Work out the finished part from the listing and answer in its coordinate system (mm). Round coordinates to 2 decimals unless told otherwise and drop trailing zeros. Order: outer loops, then holes, each group sorted by start corner. A loop starts at its lowest first (then second) coordinate and runs counter-clockwise, first axis right, second up. Notation, with made-up numbers: (-29, 7.25) -> (25, 7.25) arc R29 cw to (25, 37.25) -> close; hole circle Ø7 at (41, 0.5). An arc over 180 degrees is marked (long way). Use a Markdown table: item, result. Add a question column.
Item 1: Find the intervals of material crossed by L1, parallel to Z at x = 9, y = 1.85; L2, parallel to X at y = 0.75, z = 5.5; L3, parallel to X at y = -1.1, z = -5, in increasing order. Write a range as [from, to].
Item 2: A cutting plane is placed at D-D, the plane x = -34.7. Determine the outline of the cut face in (y, z), plus the area to 3 significant figures.
Item 3: A cutting plane is placed at A-A, the plane x = -23. Determine the outline of the cut face in (y, z).
Item 4: A cutting plane is placed at B-B, the plane z = 5. Determine the outline of the cut face in (x, y), plus the area to 3 significant figures.
Item 5: A cutting plane is placed at C-C, the plane z = -17.5. Determine the outline of the cut face in (x, y), plus the area to 3 significant figures.
Item 6: Flat-ended cylindrical pins translate along their axes: P1, Ø0.9, axis at y = -1, z = -15.5, coming from the -X side; P2, Ø1.5, axis at y = -1, z = -28, coming from the -X side; P3, Ø2, axis at x = 19, y = -1, coming from the -Z side. Find the tip coordinate at first contact, or state that the pin passes through.
from build123d import *

# Parameters (mm, degrees)
ESTRUSIONE_ESTRUSIONE1_DEPTH = 2
CORTAR_EXTRUIR4_DEPTH        = 10
CROQUIS2_R                   = 2
CROQUIS2_W                   = 40.7
CROQUIS2_H                   = 20
CORTAR_EXTRUIR5_DEPTH        = 59.660037504


with BuildPart() as part:
    # Schizzo1 → Estrusione-Estrusione1 (new, symmetric)
    with BuildSketch(Plane(origin=(0, 0, 0), x_dir=(1, 0, 0), z_dir=(0, 1, 0))):
        with BuildLine():
            Line((-25, 37.416573868), (-25, 27.25))
            Line((-25, 27.25), (25, 27.25))
            Line((25, 27.25), (25, 37.416573868))
            ThreePointArc((25, 37.416573868), (45, 0), (25, -37.416573868))
            Line((25, -37.416573868), (25, -27.25))
            Line((25, -27.25), (-25, -27.25))
            Line((-25, -27.25), (-25, -37.416573868))
            ThreePointArc((-25, -37.416573868), (-45, 0), (-25, 37.416573868))
        make_face()
    extrude(amount=ESTRUSIONE_ESTRUSIONE1_DEPTH, both=True)

    # Croquis1 → Cortar-Extruir4 (cut)
    with BuildSketch(Plane.XZ.offset(2)):
        Polygon((-8.5, 27.25), (-11.5, 27.25), (-11.5, 19.25), (-12.75, 19.25), (-12.75, 16.25), (-11.5, 16.25), (-11.5, 13.25), (-8.5, 13.25), (-8.5, 16.25), (-7.25, 16.25), (-7.25, 19.25), (-8.5, 19.25), align=None)
        Polygon((11.5, 27.25), (8.5, 27.25), (8.5, 19.25), (7.25, 19.25), (7.25, 16.25), (8.5, 16.25), (8.5, 13.25), (11.5, 13.25), (11.5, 16.25), (12.75, 16.25), (12.75, 19.25), (11.5, 19.25), align=None)
        Polygon((8.5, -13.25), (8.5, -16.25), (7.25, -16.25), (7.25, -19.25), (8.5, -19.25), (8.5, -27.25), (11.5, -27.25), (11.5, -19.25), (12.75, -19.25), (12.75, -16.25), (11.5, -16.25), (11.5, -13.25), align=None)
        Polygon((-11.5, -13.25), (-11.5, -16.25), (-12.75, -16.25), (-12.75, -19.25), (-11.5, -19.25), (-11.5, -27.25), (-8.5, -27.25), (-8.5, -19.25), (-7.25, -19.25), (-7.25, -16.25), (-8.5, -16.25), (-8.5, -13.25), align=None)
    extrude(amount=-CORTAR_EXTRUIR4_DEPTH, mode=Mode.SUBTRACT)

    # Croquis2 → Cortar-Extruir5 (cut, through all)
    with BuildSketch(Plane(origin=(0, 2, 0), x_dir=(1, 0, 0), z_dir=(0, 1, 0))):
        with Locations(Location((-34.7, 5, 0), (0, 0, 270))):
            Circle(CROQUIS2_R)
        with Locations(Location((-34.7, -5, 0), (0, 0, 270))):
            Circle(CROQUIS2_R)
        with Locations(Location((14, 5, 0), (0, 0, 270))):
            Circle(CROQUIS2_R)
        with Locations(Location((14, -5, 0), (0, 0, 270))):
            Circle(CROQUIS2_R)
        with Locations(Location((0, 21.25, 0), (0, 0, 270))):
            Circle(CROQUIS2_R)
        with Locations(Location((0, -21.25, 0), (0, 0, 270))):
            Circle(CROQUIS2_R)
        with Locations((-10.35, 0)):
            Rectangle(CROQUIS2_W, CROQUIS2_H)
    extrude(amount=-CORTAR_EXTRUIR5_DEPTH, mode=Mode.SUBTRACT)


solid = part.part
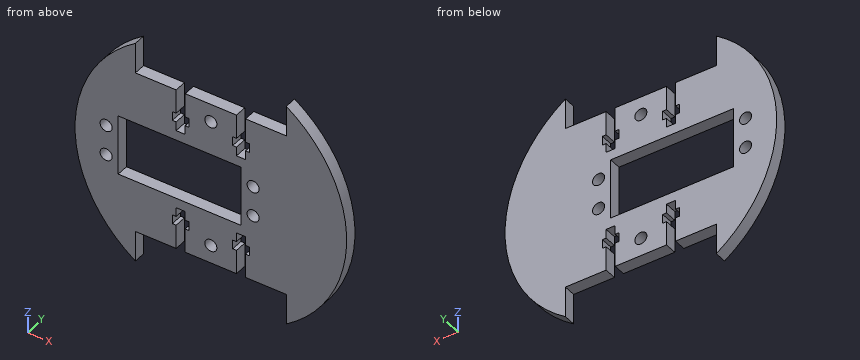
Reported:
| question | item | result |
|---|---|---|
| 1 | L1 | [-13.25, -10], [10, 13.25] |
| 1 | L2 | [-44.66, -36.64], [-32.76, -30.7], [10, 12.06], [15.94, 44.66] |
| 1 | L3 | [-44.72, -36.7], [-32.7, -30.7], [10, 12], [16, 44.72] |
| 2 | outline | (-2, -28.65) -> (2, -28.65) -> (2, -7) -> (-2, -7) -> close; (-2, -3) -> (2, -3) -> (2, 3) -> (-2, 3) -> close; (-2, 7) -> (2, 7) -> (2, 28.65) -> (-2, 28.65) -> close |
| 2 | area | 197 mm² |
| 3 | outline | (-2, -27.25) -> (2, -27.25) -> (2, -10) -> (-2, -10) -> close; (-2, 10) -> (2, 10) -> (2, 27.25) -> (-2, 27.25) -> close |
| 4 | outline | (-44.72, -2) -> (-36.7, -2) -> (-36.7, 2) -> (-44.72, 2) -> close; (-32.7, -2) -> (-30.7, -2) -> (-30.7, 2) -> (-32.7, 2) -> close; (10, -2) -> (12, -2) -> (12, 2) -> (10, 2) -> close; (16, -2) -> (44.72, -2) -> (44.72, 2) -> (16, 2) -> close |
| 4 | area | 163 mm² |
| 5 | outline | (-41.46, -2) -> (-12.75, -2) -> (-12.75, 2) -> (-41.46, 2) -> close; (-7.25, -2) -> (7.25, -2) -> (7.25, 2) -> (-7.25, 2) -> close; (12.75, -2) -> (41.46, -2) -> (41.46, 2) -> (12.75, 2) -> close |
| 5 | area | 288 mm² |
| 6 | P1 | x = -42.41 |
| 6 | P2 | x = -35.81 |
| 6 | P3 | z = -27.25 |
